```python
from build123d import *

# Parameters (mm, degrees)
F0_R      = 12.7
F1_DEPTH  = 50.8
F2_R      = 5.08
F3_SIZE   = 5.08
F1_FACE_R = 7.62
F4_DEPTH  = 25.4


with BuildPart() as f1:
    # F0 (on Top) → F1 (new body)
    with BuildSketch(Plane.XY):
        Circle(F0_R)
    extrude(amount=F1_DEPTH)

    # F2
    f2_edges = [f1.edges().sort_by_distance(p)[0] for p in [
        (-12.7, 0, 50.8),
    ]]
    fillet(f2_edges, radius=F2_R)

    # F3
    f3_edges = [f1.edges().sort_by_distance(p)[0] for p in [
        (-12.7, 0, 0),
    ]]
    chamfer(f3_edges, length=F3_SIZE)

    # F1_face (on face) → F4 (cut)
    with BuildSketch(Plane.XY.offset(50.8)):
        Circle(F1_FACE_R)
    extrude(amount=-F4_DEPTH, mode=Mode.SUBTRACT)


solid = f1.part
```
Geometry check sheet. Reference: the model listing, model coordinates, mm. A direction names the side the tool comes from. Coordinates: 2 decimals unless noted, no trailing zeros. Order: outer loops, then holes, each group sorted by start corner. A loop starts at its lowest first (then second) coordinate and runs counter-clockwise, first axis right, second up. Notation, with made-up numbers: (85, 1) - (116, 1) arc R9 ccw to (116, 13) - close; hole circle Ø6 at (53, 86.25). An arc over 180 degrees is marked (long way). Use one line per item in the form item = value.
1. Section check C-C (z = 21.5). Record the boundary of the cut face in (x, y), then the cut area to 3 significant figures.
Here are the results:
outline = circle Ø25.4 at (0, 0)
area = 507 mm²
2. Scan lines: line 1 (Y direction, x = 0, z = 42.75); line 2 (Z direction, x = 1.5, y = -1); line 3 (X direction, y = -5.5, z = 37.5). Record each from-to range of solid material in increasing order.
Here are the results:
line_1 = -12.7 to -7.62, 7.62 to 12.7
line_2 = 0 to 25.4
line_3 = -11.45 to -5.27, 5.27 to 11.45
3. Access from +Z, -Z, +X, -X, +Y, -Y to the whole of each face (thin tool, end or side, straight path). Record for faces 1 (the face through (-1.65, -7.44, 38.28)), 2 (the face through (-7.86, 0.35, 0.25)).
Here are the results:
face_1 = +Z
face_2 = -Z
4. Draft check along Y on faces 3 (the face through (0, 0, 0)), 4 (the face through (0, 0, 25.4)), 5 (the face through (-2.75, -12.4, 25.12)). Enter one of: pulls with the +Y half, pulls with the -Y half, needs draft (parallel to the pull), parting line crosses it, or undercut.
Here are the results:
face_3 = needs draft
face_4 = undercut
face_5 = parting line crosses it
5. Section check D-D (z = 42.5). Record the boundary of the cut face in (x, y), then the cut area to 3 significant figures.
Here are the results:
outline = circle Ø25.4 at (0, 0); hole circle Ø15.24 at (0, 0)
area = 324 mm²
6. Gauge pin test, flat ends, axial feed: pin 1 (1 mm diameter, centred on x = 7.5, z = 29.5, fed in from +Y); pin 2 (12 mm diameter, centred on y = -7, z = 21, fed in from +X); pin 3 (13.5 mm diameter, centred on x = 0, y = 0, fed in from +Z). Record the tip position at first contact, or that the pin passes through.
Here are the results:
pin_1 = 10.6
pin_2 = 12.66
pin_3 = 25.4
7. Section check A-A (y = 0). Record the boundary of the cut face in (x, z).
Here are the results:
outline = (-12.7, 5.08) - (-7.62, 0) - (7.62, 0) - (12.7, 5.08) - (12.7, 45.72) arc R5.08 ccw to (7.62, 50.8) - (7.62, 25.4) - (-7.62, 25.4) - (-7.62, 50.8) arc R5.08 ccw to (-12.7, 45.72) - close
